from build123d import *

# Parameters (mm, degrees)
F1_DEPTH = 85
F2_R     = 4.99999


# Not quite as in the source:
# - a fillet or chamfer is up to 0.001 mm smaller than in the source, because OpenCascade refuses the exact size


with BuildPart() as f1:
    # F0 (on Front) → F1 (new body, symmetric)
    with BuildSketch(Plane.XZ):
        Polygon((15, 15), (-15, 15), (-15, 10), (10, 10), (10, -15), (15, -15), align=None)
    extrude(amount=F1_DEPTH, both=True)

    # F2 (radius 5 in the source; OpenCascade refuses exactly that, so slightly less here)
    f2_edges = [f1.edges().sort_by_distance(p)[0] for p in [
        (-15, 0, 15),
        (15, 0, 15),
        (15, 0, -15),
    ]]
    fillet(f2_edges, radius=F2_R)


solid = f1.part
Part model, mm, in its own coordinate system. A direction names the side the tool comes from. Coordinates: 2 decimals unless noted, no trailing zeros. Order: outer loops, then holes, each group sorted by start corner. A loop starts at its lowest first (then second) coordinate and runs counter-clockwise, first axis right, second up. Notation, with made-up numbers: M 19,54 L 65,54 A28 ccw 65,73 Z; hole C -1,-27 d9. An arc over 180 degrees is marked long. Use a Markdown table: item, result.
(1) Tool access for faces 1 (the cylindrical face through (14, 1, -13)), 2 (the flat face through (10, -1, -2)): list every direction of +Z, -Z, +X, -X, +Y, -Y with a clear straight run to the whole face (end or side of a thin tool).
A:
| item | result |
|---|---|
| face 1 | -Z, +X, +Y, -Y |
| face 2 | -Z, -X, +Y, -Y |
(2) Probe L1, parallel to X at y = 51, z = -6; L2, parallel to Z at x = 10.25, y = -32. List the from-to ranges inside material, lowest first.
A:
| item | result |
|---|---|
| L1 | x = 10 to 15 |
| L2 | z = -14.99 to 14.99 |
(3) Cut at B-B on x = 6. Write the cut outline in (y, z), then the cut area to 3 significant figures.
A:
| item | result |
|---|---|
| outline | M -85,10 L 85,10 L 85,15 L -85,15 Z |
| area | 850 mm^2 |
(4) Cut at C-C on z = -4. Write the cut outline in (x, y), then the cut area to 3 significant figures.
A:
| item | result |
|---|---|
| outline | M 10,-85 L 15,-85 L 15,85 L 10,85 Z |
| area | 850 mm^2 |
(5) Flat gauge pins, fed straight in: pin 1 (7.5 mm diameter, centred on y = 32, z = -6, fed in from -X); pin 2 (10 mm diameter, centred on x = -9.5, y = -25, fed in from -Z); pin 3 (3 mm diameter, centred on x = 7, z = -8.5, fed in from +Y). Where does each tip first touch, or does it go through?
A:
| item | result |
|---|---|
| pin 1 | stops at x = 10 |
| pin 2 | stops at z = 10 |
| pin 3 | passes through |
